Verification items for the finished model (mm, model axes). A direction names the side the tool comes from. Round coordinates to 2 decimals unless told otherwise and drop trailing zeros. Write each loop counter-clockwise with the first axis right and the second up, starting at its lowest first coordinate (ties: lowest second). Pieces come first, ordered by that corner, then holes. Notation, with made-up numbers: (42, 2.25) - (58, 2.25) arc R14 ccw to (58, 25.25) - close; hole circle Ø10 at (-11.5, 9). An arc over 180 degrees is marked (long way). Answer as a JSON object with one key per item and string values. Group by question number.
1) Thickness scan on line 1 (Y direction, x = -3, z = 1.75); line 2 (X direction, y = 52, z = 5). Record the ranges inside material, lowest first.
2) Set-up check for faces 5 (the flat face through (-14, 10, 5)), 6 (the flat face through (-32, 14, 5)), 7 (the cylindrical face through (-0.6, 65.43, 4.93)), 8 (the cylindrical face through (-27.4, 10.57, 4.93)): record each of +Z, -Z, +X, -X, +Y, -Y from which the full face is reachable in a straight line by a thin tool's end or side.
3) Mould release check, pull along Y, two halves, no side actions. Record for faces 1 (the flat face through (-8, 73, 5)), 2 (the flat face through (0, 38, 5)), 3 (the cylindrical face through (-28.43, 13.55, 4.93)), 4 (the cylindrical face through (-0.57, 10.6, 4.93)): +Y half, -Y half, draft (parallel to the pull), parting line (faces both ways), or undercut.
4) Section check C-C (y = 39.5). Enter the section's corners in (x, z).
5) Section check A-A (z = 3). Enter the section's corners in (x, y), then the cut area to 3 significant figures.
6) Go/stop test with flat-tipped pins: pin 1 Ø3.5 at (x, z) = (-3.5, 5) entering from -Y; pin 2 Ø4 at (y, z) = (66.5, 7.5) entering from -X; pin 3 Ø1 at (y, z) = (8, 2) entering from +X; pin 4 Ø3 at (x, z) = (-12, 6) entering from +Y. Record where each tip stops, or that it passes through.
7) Section check B-B (y = 11). Enter the section's corners in (x, z), then the cut area to 3 significant figures.
```python
from build123d import *

# Parameters (mm, degrees)
EXTRUDE_1_DEPTH = 10


with BuildPart() as part:
    # 草图1 → 凸台-拉伸1 (new body)
    with BuildSketch(Plane.XY):
        with BuildLine():
            Line((-6.5, 66), (-2, 66))
            ThreePointArc((-2, 66), (-0.585786438, 65.414213562), (0, 64))
            Line((0, 64), (0, 16))
            Line((0, 16), (0, 12))
            ThreePointArc((0, 12), (-0.585786438, 10.585786438), (-2, 10))
            Line((-2, 10), (-6.5, 10))
            Line((-6.5, 10), (-26, 10))
            ThreePointArc((-26, 10), (-27.414213562, 10.585786438), (-28, 12))
            Line((-28, 12), (-28, 12.5))
            ThreePointArc((-28, 12.5), (-28.439339828, 13.560660172), (-29.5, 14))
            Line((-29.5, 14), (-34, 14))
            ThreePointArc((-34, 14), (-35.414213562, 13.414213562), (-36, 12))
            Line((-36, 12), (-36, 2))
            ThreePointArc((-36, 2), (-35.414213562, 0.585786438), (-34, 0))
            Line((-34, 0), (0, 0))
            ThreePointArc((0, 0), (7.071067812, 2.928932188), (10, 10))
            Line((10, 10), (10, 75))
            ThreePointArc((10, 75), (8.535533906, 78.535533906), (5, 80))
            Line((5, 80), (-6.5, 80))
            ThreePointArc((-6.5, 80), (-7.560660172, 79.560660172), (-8, 78.5))
            Line((-8, 78.5), (-8, 67.5))
            ThreePointArc((-8, 67.5), (-7.560660172, 66.439339828), (-6.5, 66))
        make_face()
    extrude(amount=EXTRUDE_1_DEPTH)


solid = part.part
```
Returned:
{
 "1": {"line 1": "0 to 10, 66 to 80", "line 2": "0 to 10"},
 "2": {"face 5": "+Z, -Z", "face 6": "+Z, -Z, -X, +Y", "face 7": "+Z, -Z, -X", "face 8": "+Z, -Z, +Y"},
 "3": {"face 1": "draft", "face 2": "undercut", "face 3": "+Y half", "face 4": "undercut"},
 "4": {"outline": "(0, 0) - (10, 0) - (10, 10) - (0, 10) - close"},
 "5": {"outline": "(-36, 2) arc R2 ccw to (-34, 0) - (0, 0) arc R10 ccw to (10, 10) - (10, 75) arc R5 ccw to (5, 80) - (-6.5, 80) arc R1.5 ccw to (-8, 78.5) - (-8, 67.5) arc R1.5 ccw to (-6.5, 66) - (-2, 66) arc R2 cw to (0, 64) - (0, 12) arc R2 cw to (-2, 10) - (-26, 10) arc R2 cw to (-28, 12) - (-28, 12.5) arc R1.5 ccw to (-29.5, 14) - (-34, 14) arc R2 ccw to (-36, 12) - close", "area": "1,280 mm2"},
 "6": {"pin 1": "y = 0", "pin 2": "x = -8", "pin 3": "x = 9.89", "pin 4": "y = 10"},
 "7": {"outline": "(-36, 0) - (-27.73, 0) - (-27.73, 10) - (-36, 10) - close; (-0.27, 0) - (10, 0) - (10, 10) - (-0.27, 10) - close", "area": "185 mm2"}
}
